from build123d import *

# Parameters (mm, degrees)
F0_R     = 4.0005
F1_DEPTH = 6.985
F2_R     = 2.8575
F3_DEPTH = 5.715


with BuildPart() as f1:
    # F0 (on Front) → F1 (new body, symmetric)
    with BuildSketch(Plane.XZ):
        Polygon((8.89, 13.335), (-8.89, 13.335), (-8.89, -13.462), (-20.6375, -13.462), (-20.6375, -19.177), (20.6375, -19.177), (20.6375, -13.462), (8.89, -13.462), align=None)
        Circle(F0_R, mode=Mode.SUBTRACT)
    extrude(amount=F1_DEPTH, both=True)

    # F2 (on face) → F3 (cut, through all)
    with BuildSketch(Plane(origin=(0, 0, -19.177), x_dir=(1, 0, 0), z_dir=(0, 0, -1))):
        with Locations((-15.5575, 0)):
            Circle(F2_R)
        with Locations((15.5575, 0)):
            Circle(F2_R)
    extrude(amount=-F3_DEPTH, mode=Mode.SUBTRACT)


solid = f1.part
For this review, take the finished solid that the model builds, in its own axes (mm). A direction names the side the tool comes from. Give positions to 0.01 mm unless a question says otherwise; leave off trailing zeros. Loops run counter-clockwise (first coordinate to the right, second up) from the corner with the lowest first, then second, coordinate; pieces in that order, holes last. Notation, with made-up numbers: M 15,82 L 43,82 A14 ccw 43,104 Z; hole C 36,-11.75 d8. An arc over 180 degrees is marked long. Put each result on its own line as item: value. Start each with the question number.
(1) Add section A-A, the plane y = 0. Write out the cut boundary in (x, z) (1 decimal).
(2) Add section D-D, the plane y = 4. Write out the cut boundary in (x, z) (1 decimal), then the cut area to 3 significant figures.
(3) For pin 1 (3 mm diameter, centred on y = -5, z = -0.5, fed in from -X); pin 2 (5 mm diameter, centred on x = 0, z = 0, fed in from +Y); pin 3 (7 mm diameter, centred on y = -3, z = -4, fed in from +X), all flat-tipped, find the tip position at first contact; note any pin that passes through.
(4) Wall thickness on L1, parallel to X at y = 0, z = -15.35 (1 decimal); L2, parallel to Z at x = 15, y = 6; L3, parallel to X at y = -2.25, z = -18: over which ranges is each line inside the solid? List them lowest first.
(5) Add section C-C, the plane z = 0. Write out the cut boundary in (x, y) (1 decimal).
(6) The part is to be moulded in two halves that separate along Y. For faces 4 (the flat face through (0, 6.985, -6)), 5 (the flat face through (0, 0, -19.177)), 6 (the cylindrical face through (12.7, -0.1, -16.4)), say which applies: +Y half, -Y half, draft (parallel to the pull), parting line (faces both ways), or undercut.
(7) Add section B-B, the plane x = 0. Write out the cut boundary in (y, z) (1 decimal).
(8) Machinability: for faces 1 (the flat face through (-8.89, 0, 0)), 2 (the flat face through (8.89, 0, 0)), 3 (the flat face through (0, -6.985, -6)), which of the approach directions +Z, -Z, +X, -X, +Y, -Y give a long, thin tool a straight path to every point of the face, cutting with its end or side? Answer none if there is none.
Result:
1. outline: M -20.6,-19.2 L -18.4,-19.2 L -18.4,-13.5 L -20.6,-13.5 Z; M -12.7,-19.2 L 12.7,-19.2 L 12.7,-13.5 L 8.9,-13.5 L 8.9,13.3 L -8.9,13.3 L -8.9,-13.5 L -12.7,-13.5 Z; M 18.4,-19.2 L 20.6,-19.2 L 20.6,-13.5 L 18.4,-13.5 Z; hole C 0,0 d8
2. outline: M -20.6,-19.2 L 20.6,-19.2 L 20.6,-13.5 L 8.9,-13.5 L 8.9,13.3 L -8.9,13.3 L -8.9,-13.5 L -20.6,-13.5 Z; hole C 0,0 d8
2. area: 662 mm^2
3. pin 1: stops at x = -8.89
3. pin 2: passes through
3. pin 3: stops at x = 8.89
4. L1: x = -20.6 to -18.4, -12.7 to 12.7, 18.4 to 20.6
4. L2: z = -19.18 to -13.46
4. L3: x = -20.64 to -17.32, -13.8 to 13.8, 17.32 to 20.64
5. outline: M -8.9,-7 L -4,-7 L -4,7 L -8.9,7 Z; M 4,-7 L 8.9,-7 L 8.9,7 L 4,7 Z
6. face 4: +Y half
6. face 5: draft
6. face 6: undercut
7. outline: M -7,-19.2 L 7,-19.2 L 7,-4 L -7,-4 Z; M -7,4 L 7,4 L 7,13.3 L -7,13.3 Z
8. face 1: +Z, -X, +Y, -Y
8. face 2: +Z, +X, +Y, -Y
8. face 3: +Z, -Z, +X, -X, -Y
